For this review, take the finished solid that the model builds, in its own axes (mm). A direction names the side the tool comes from. Round coordinates to 2 decimals unless told otherwise and drop trailing zeros. Order: outer loops, then holes, each group sorted by start corner. A loop starts at its lowest first (then second) coordinate and runs counter-clockwise, first axis right, second up. Notation, with made-up numbers: (38, 38.5) -> (47, 38.5) arc R29 cw to (47, 65.5) -> close; hole circle Ø1 at (34.25, 20.5). An arc over 180 degrees is marked (long way). Answer in a Markdown table with one row per item.
```python
from build123d import *

# Parameters (mm, degrees)
CUT_EXTRUDE_1_DEPTH      = 0.5
PATTERN_CIRCULAR_1_COUNT = 12
CHAMFER_1_SIZE           = 1


with BuildPart() as part:
    # 草图1 → 旋转1 (revolve)
    with BuildSketch(Plane(origin=(0, 0, 0), x_dir=(-1, 0, 0), z_dir=(0, 0, -1)), mode=Mode.PRIVATE) as revolve_1_sk:
        Polygon((-7, 46.5), (-9.5, 46.5), (-9.5, 47.5), (-12, 47.5), (-12, 45), (0, 45), (0, 52.5), (-12, 52.5), (-12, 50.5), (-7, 50.5), align=None)
    revolve(revolve_1_sk.sketch.rotate(Axis((17.910447761, 0, 0), (-1, 0, 0)), 270), axis=Axis((17.910447761, 0, 0), (-1, 0, 0)))

    # 草图2 → 切除-拉伸1 (cut)
    with BuildSketch(Plane.ZY):
        with BuildLine():
            Line((-47.434902901, -2.485957922), (-50.430791505, -2.64296579))
            ThreePointArc((-50.430791505, -2.64296579), (-50.5, 0), (-50.430791505, 2.64296579))
            Line((-50.430791505, 2.64296579), (-47.434902901, 2.485957922))
            ThreePointArc((-47.434902901, 2.485957922), (-47.5, 0), (-47.434902901, -2.485957922))
        make_face()
    cut_extrude_1 = extrude(amount=-CUT_EXTRUDE_1_DEPTH, mode=Mode.SUBTRACT)

    # 阵列(圆周)1: 切除-拉伸1 ×12 about axis
    pattern_circular_1_axis = Axis((0, 0, 0), (1, 0, 0))
    for i in range(1, PATTERN_CIRCULAR_1_COUNT):
        add(cut_extrude_1.rotate(pattern_circular_1_axis, i * 360 / PATTERN_CIRCULAR_1_COUNT), mode=Mode.SUBTRACT)

    # 倒角1
    chamfer_1_edges = [part.edges().sort_by_distance(p)[0] for p in [
        (0, 0, -45),
        (12, 0, -45),
    ]]
    chamfer(chamfer_1_edges, length=CHAMFER_1_SIZE)


solid = part.part
```
Q1. Take a section at C-C, the plane x = 5. Write out the cut boundary in (y, z).
Answer key:
| item | result |
|---|---|
| outline | circle Ø105 at (0, 0); hole circle Ø90 at (0, 0) |
Q2. Tool access review of faces 4 (the face through (7, -15, 45)), 5 (the face through (0.5, -49, 0)): name each direction out of +Z, -Z, +X, -X, +Y, -Y from which nothing blocks a thin tool from reaching the whole face with its end or side.
Answer key:
| item | result |
|---|---|
| face 4 | none |
| face 5 | -X |
Q3. The part is to be moulded in two halves that separate along Y. For faces 1 (the face through (0.5, 0, -49)), 2 (the face through (0, -46.4, 0.2)), 3 (the face through (6.084, 15.77, 50.076)), say which applies: +Y half, -Y half, draft (parallel to the pull), parting line (faces both ways), or undercut.
Answer key:
| item | result |
|---|---|
| face 1 | undercut |
| face 2 | draft |
| face 3 | parting line |
Q4. Clearance check with flat-ended pins moving along their axes: pin 1 Ø2 at (x, z) = (10, 1) entering from +Y; pin 2 Ø5 at (x, y) = (7, -33) entering from +Z; pin 3 Ø5 at (x, y) = (5, -28) entering from -Z. State where each tip first meets the part, or that it passes through.
Answer key:
| item | result |
|---|---|
| pin 1 | stops at y = 52.5 |
| pin 2 | stops at z = 42.73 |
| pin 3 | stops at z = -45.89 |
Q5. To check wall thickness, follow probe 1 along Y at (x, z) = (8.55, 0); probe 2 along Z at (x, y) = (11, -1); probe 3 along X at (y, z) = (22, -41). State the ranges of each line that lie inside material, in increasing order.
Answer key:
| item | result |
|---|---|
| probe 1 | y = -52.5 to -50.5, -46.5 to -45, 45 to 46.5, 50.5 to 52.5 |
| probe 2 | z = -52.49 to -50.49, -47.49 to -44.99, 44.99 to 47.49, 50.49 to 52.49 |
| probe 3 | x = 0 to 7, 9.5 to 12 |
